from build123d import *

# Parameters (mm, degrees)
SKETCH1_R           = 5
BOSS_EXTRUDE1_DEPTH = 2.2


with BuildPart() as part:
    # Sketch1 → Boss-Extrude1 (new body)
    with BuildSketch(Plane(origin=(0, 0, 0), x_dir=(1, 0, 0), z_dir=(0, 1, 0))):
        Polygon((-145.195425431, -13.597712716), (-145.195425431, -11.597712716), (-153.195425431, -11.597712716), (-153.195425431, -13.597712716), (-161.195425431, -13.597712716), (-161.195425431, -36.597712716), (-153.195425431, -36.597712716), (-153.195425431, -34.597712716), (-145.195425431, -34.597712716), (-145.195425431, -36.597712716), (-137.195425431, -36.597712716), (-137.195425431, -30.597712716), (-138.695425431, -30.597712716), (-138.695425431, -22.597712716), (-137.195425431, -22.597712716), (-137.195425431, -16.597712716), (-137.195425431, -13.597712716), align=None)
        with Locations(Location((-149.195425431, -24.097712716, 0), (0, 0, 270))):
            Circle(SKETCH1_R, mode=Mode.SUBTRACT)
    extrude(amount=BOSS_EXTRUDE1_DEPTH)


solid = part.part
Geometry: final body of the model. Coordinates: model frame, mm. A direction names the side the tool comes from. Give positions to 0.01 mm unless a question says otherwise; leave off trailing zeros. Loops run counter-clockwise (first coordinate to the right, second up) from the corner with the lowest first, then second, coordinate; pieces in that order, holes last. Notation, with made-up numbers: (87.5, 26.5) - (120.5, 26.5) arc R30 ccw to (120.5, 57.5) - close; hole circle Ø4 at (35, 76.5). An arc over 180 degrees is marked (long way). Answer as CSV lines item,"result". Start each with the question number.
1. Pin query (flat end, axial travel): P1, Ø1, axis at y = 1, z = 13, coming from the +X side; P2, Ø0.7, axis at x = -140.5, y = 1, coming from the -Z side; P3, Ø1.1, axis at x = -147.5, y = 1.5, coming from the +Z side. Return the tip coordinate at first contact, or that it passes through.
2. Section B-B, the plane z = 20. Return loops of the section in (x, y), plus the area to 3 significant figures.
3. Draft query along Z for faces 6 (the face through (-157, 1, 13.598)), 7 (the face through (-145.195, 1, 13)), 8 (the face through (-138.695, 1, 27)). Return one class per face: released by +Z, released by -Z, zero draft, split by the parting line, or undercut.
4. Section D-D, the plane z = 30.25. Return loops of the section in (x, y), plus the area to 3 significant figures.
5. Section C-C, the plane y = 1.35. Return loops of the section in (x, z), plus the area to 3 significant figures.
6. Ray query, L1, parallel to Z at x = -149.25, y = 0.7; L2, parallel to Z at x = -155.5, y = 0.65; L3, parallel to X at y = 1.4, z = 25. Return the intervals inside material, ascending.
7. Section A-A, the plane x = -144.75. Return loops of the section in (y, z).
8. Reachability of faces 1 (the face through (-137.195, 1, 34)), 2 (the face through (-141, 1, 13.598)), 3 (the face through (-138, 1, 22.598)), 4 (the face through (-153.195, 1, 36)), 5 (the face through (-153.195, 1, 13)) from +Z, -Z, +X, -X, +Y, -Y: full face, straight path, thin tool, end or side. Return the list, or none.
Answers:
1,P1,"stops at x = -145.2"
1,P2,"stops at z = 13.6"
1,P3,"stops at z = 34.6"
2,outline,"(-161.2, 0) - (-152.06, 0) - (-152.06, 2.2) - (-161.2, 2.2) - close; (-146.33, 0) - (-137.2, 0) - (-137.2, 2.2) - (-146.33, 2.2) - close"
2,area,"40.2 mm2"
3,face 6,"released by -Z"
3,face 7,"zero draft"
3,face 8,"undercut"
4,outline,"(-161.2, 0) - (-138.7, 0) - (-138.7, 2.2) - (-161.2, 2.2) - close"
4,area,"49.5 mm2"
5,outline,"(-161.2, 13.6) - (-153.2, 13.6) - (-153.2, 11.6) - (-145.2, 11.6) - (-145.2, 13.6) - (-137.2, 13.6) - (-137.2, 22.6) - (-138.7, 22.6) - (-138.7, 30.6) - (-137.2, 30.6) - (-137.2, 36.6) - (-145.2, 36.6) - (-145.2, 34.6) - (-153.2, 34.6) - (-153.2, 36.6) - (-161.2, 36.6) - close; hole circle Ø10 at (-149.2, 24.1)"
5,area,"461 mm2"
6,L1,"z = 11.6 to 19.1, 29.1 to 34.6"
6,L2,"z = 13.6 to 36.6"
6,L3,"x = -161.2 to -154.11, -144.28 to -138.7"
7,outline,"(0, 13.6) - (2.2, 13.6) - (2.2, 21.81) - (0, 21.81) - close; (0, 26.39) - (2.2, 26.39) - (2.2, 36.6) - (0, 36.6) - close"
8,face 1,"+Z, -Z, +X, +Y, -Y"
8,face 2,"-Z, +X, +Y, -Y"
8,face 3,"+X, +Y, -Y"
8,face 4,"+Z, +Y, -Y"
8,face 5,"-Z, -X, +Y, -Y"
